For this review, use the dimensioned drawing (mm, ordinates from the lowest corner) and the shaded views. Round coordinates to 2 decimals unless told otherwise and drop trailing zeros. Loops run counter-clockwise (first coordinate to the right, second up) from the corner with the lowest first, then second, coordinate; pieces in that order, holes last. Notation, with made-up numbers: (-6.75, 58.25) - (4.25, 58.25) arc R21 cw to (4.25, 74.25) - close; hole circle Ø6 at (89.5, 77). An arc over 180 degrees is marked (long way). Answer as CSV lines item,"result". Start each with the question number.
(1) Consider section A-A (y = 7). Give the boundary of the cut face in (x, z) (3 decimals), and give its area (3 significant figures).
(2) For P1, Ø4, axis at x = 113, z = 15.5, coming from the -Y side; P2, Ø1, axis at y = 15, z = 8, coming from the +X side; P3, Ø2, axis at y = 33, z = 4, coming from the -X side, all flat-tipped, find the tip position at first contact; note any pin that passes through.
(3) Wall thickness on L1, parallel to Z at x = 84, y = 51 (3 decimals); L2, parallel to Y at x = 102, z = 7; L3, parallel to X at y = 5, z = 17.25: over which ranges is each line inside the solid? List them lowest first.
(4) Consider section C-C (y = 40). Give the boundary of the cut face in (x, z) (3 decimals).
(5) Consider section D-D (x = 104). Give the boundary of the cut face in (y, z) (3 decimals), and give its area (3 significant figures).
(6) Mouldability with a two-part tool opening along X and no side actions: class the marked faces 1, 2, 3 and 4 as released by +X, released by -X, zero draft, split by the parting line, or undercut.
(7) Consider section B-B (z = 3). Give the boundary of the cut face in (x, y).
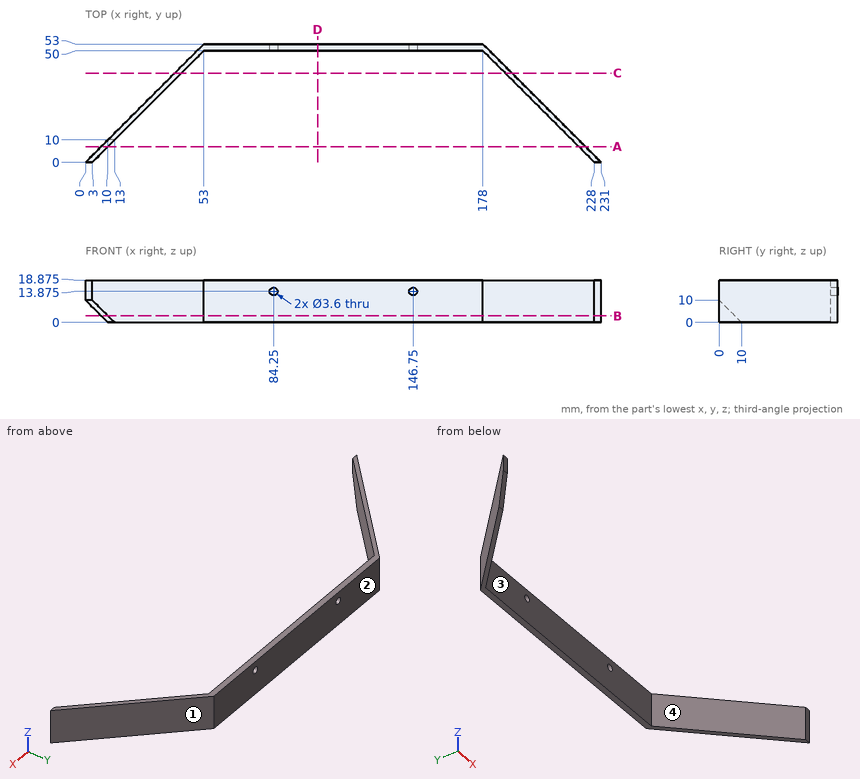
Determined:
1,outline,"(7, 3) - (10, 3) - (10, 18.875) - (7, 18.875) - close; (221, 0) - (224, 0) - (224, 18.875) - (221, 18.875) - close"
1,area,"104 mm^2"
2,P1,"stops at y = 50"
2,P2,"stops at x = 216.5"
2,P3,"stops at x = 32"
3,L1,"z = 0 to 12.092, 15.658 to 18.875"
3,L2,"y = 50 to 53"
3,L3,"x = 5 to 8, 223 to 226"
4,outline,"(40, 0) - (43, 0) - (43, 18.875) - (40, 18.875) - close; (188, 0) - (191, 0) - (191, 18.875) - (188, 18.875) - close"
5,outline,"(50, 0) - (53, 0) - (53, 18.875) - (50, 18.875) - close"
5,area,"56.6 mm^2"
6,face 1,"released by +X"
6,face 2,"zero draft"
6,face 3,"undercut"
6,face 4,"undercut"
7,outline,"(7, 7) - (10, 7) - (53, 50) - (178, 50) - (228, 0) - (231, 0) - (178, 53) - (53, 53) - close"
